Geometry: final body of the model. Coordinates: model frame, mm. A direction names the side the tool comes from. Give positions to 0.01 mm unless a question says otherwise; leave off trailing zeros. Write each loop counter-clockwise with the first axis right and the second up, starting at its lowest first coordinate (ties: lowest second). Pieces come first, ordered by that corner, then holes. Notation, with made-up numbers: (-8.5, -28.5) -> (47.5, -28.5) arc R30 ccw to (47.5, 4.5) -> close; hole circle Ø6 at (47.25, 24.25). An arc over 180 degrees is marked (long way). Answer in a Markdown table with one row per item. Add a question column.
Item 1: Access query for faces 1 (the flat face through (-27.826, 0, 17)), 2 (the flat face through (-36, -20, 17)), 3 (the flat face through (-25.826, 0, 17)). Directions: +Z, -Z, +X, -X, +Y, -Y. A direction counts if a zero-diameter tool reaches every point of the face in a straight line with its end or side. Return the directions, or none.
Item 2: Material intervals for probe 1 along Y at (x, z) = (-30, 22.5); probe 2 along X at (y, z) = (1.5, 15); probe 3 along X at (y, z) = (-17, 11.5), sorted ascending. Write a range as from..to.
Item 3: Section query C-C on x = 0. Output: boundary loops of the cut face in (y, z).
Item 4: Section query D-D on z = 9.25. Output: boundary loops of the cut face in (x, y).
Item 5: First-contact query: P1, Ø8.5, axis at x = -35.5, z = 14, coming from the +Y side; P2, Ø2.5, axis at x = 1.5, z = 1.5, coming from the -Y side; P3, Ø5.5, axis at y = 4.5, z = 3.5, coming from the +X side; P4, Ø10, axis at y = -27, z = 22, coming from the +X side. Flat tips, straight axial feed; report the tip coordinate or a pass-through.
Item 6: Section query A-A on z = 19.25. Output: boundary loops of the cut face in (x, y).
Item 7: Section query B-B on y = 0. Output: boundary loops of the cut face in (x, z).
Item 8: Draft query along Z for faces 4 (the flat face through (0, -11.543, 3)), 5 (the flat face through (-49, 0, 11)), 6 (the flat face through (10, 1, 0)). Return one class per face: +Z half, -Z half, draft (parallel to the pull), parting line (faces both ways), or undercut.
```python
from build123d import *

# Parameters (mm, degrees)
F0_R      = 50
F1_DEPTH  = 5
F3_DEPTH  = 25
F4_T      = -2
F6_W      = 10
F6_H      = 3
F7_DEPTH  = 3
F8_W      = 12.0332203805
F8_H      = 23.0855867267
F9_DEPTH  = 25
F10_R     = 50
F10_W     = 12.0332203805
F10_H     = 23.0855867267
F11_DEPTH = 5


with BuildPart() as f1:
    # F0 (on Top) → F1 (new body)
    with BuildSketch(Plane.XY):
        Circle(F0_R)
    extrude(amount=F1_DEPTH)

    # F2 (on face) → F3 (join)
    with BuildSketch(Plane.XY.offset(5)):
        with BuildLine():
            Line((-25.8257569496, 20), (-45.8257569496, 20))
            ThreePointArc((-45.8257569496, 20), (-50, 0), (-45.8257569496, -20))
            Line((-45.8257569496, -20), (-25.8257569496, -20))
            Line((-25.8257569496, -20), (-25.8257569496, 20))
        make_face()
    extrude(amount=F3_DEPTH)

    # F4
    f4_openings = [f1.faces().sort_by_distance(p)[0] for p in [
        (-37.262739, 0, 30),
    ]]
    offset(amount=F4_T, openings=f4_openings)

    # F6 (on offset) → F7 (cut)
    with BuildSketch(Plane.YZ.offset(-50)):
        with Locations((0, 9.5)):
            Rectangle(F6_W, F6_H)
    extrude(amount=F7_DEPTH, mode=Mode.SUBTRACT)

    # F8 (on face) → F9 (cut)
    with BuildSketch(Plane.XY.offset(5)):
        Rectangle(F8_W, F8_H)
    extrude(amount=-F9_DEPTH, mode=Mode.SUBTRACT)

    # F10 (on face) → F11 (join)
    with BuildSketch(Plane(origin=(0, 0, 0), x_dir=(1, 0, 0), z_dir=(0, 0, -1))):
        Circle(F10_R)
        Rectangle(F10_W, F10_H, mode=Mode.SUBTRACT)
    extrude(amount=-F11_DEPTH)


solid = f1.part
```
Findings below:
| question | item | result |
|---|---|---|
| 1 | face 1 | +Z |
| 1 | face 2 | +Z, +X, -X, -Y |
| 1 | face 3 | +Z, +X, +Y, -Y |
| 2 | probe 1 | y = -20..-18, 18..20 |
| 2 | probe 2 | x = -49.98..-47.98, -27.83..-25.83 |
| 2 | probe 3 | x = -47.02..-44.89, -27.83..-25.83 |
| 3 | outline | (-50, 0) -> (-11.54, 0) -> (-11.54, 5) -> (-50, 5) -> close; (11.54, 0) -> (50, 0) -> (50, 5) -> (11.54, 5) -> close |
| 4 | outline | (-49.75, -5) arc R50 ccw to (-45.83, -20) -> (-25.83, -20) -> (-25.83, 20) -> (-45.83, 20) arc R50 ccw to (-49.75, 5) -> (-47.74, 5) arc R48 cw to (-44.5, 18) -> (-27.83, 18) -> (-27.83, -18) -> (-44.5, -18) arc R48 cw to (-47.74, -5) -> close |
| 5 | P1 | stops at y = 20 |
| 5 | P2 | stops at y = -50 |
| 5 | P3 | stops at x = 49.97 |
| 5 | P4 | passes through |
| 6 | outline | (-45.83, -20) -> (-25.83, -20) -> (-25.83, 20) -> (-45.83, 20) arc R50 ccw to start; hole (-44.5, -18) -> (-27.83, -18) -> (-27.83, 18) -> (-44.5, 18) arc R48 ccw to start |
| 7 | outline | (-50, 0) -> (-6.02, 0) -> (-6.02, 5) -> (-25.83, 5) -> (-25.83, 30) -> (-27.83, 30) -> (-27.83, 5) -> (-48, 5) -> (-48, 8) -> (-50, 8) -> close; (-50, 11) -> (-48, 11) -> (-48, 30) -> (-50, 30) -> close; (6.02, 0) -> (50, 0) -> (50, 5) -> (6.02, 5) -> close |
| 8 | face 4 | draft |
| 8 | face 5 | undercut |
| 8 | face 6 | -Z half |
